For this review, take the finished solid that the model builds, in its own axes (mm). Face numbers are marked on the shaded views. A direction names the side the tool comes from. Round coordinates to 2 decimals unless told otherwise and drop trailing zeros. Loops run counter-clockwise (first coordinate to the right, second up) from the corner with the lowest first, then second, coordinate; pieces in that order, holes last. Notation, with made-up numbers: (19, 77) -> (39, 77) arc R30 ccw to (39, 109) -> close; hole circle Ø2 at (-21.5, 37). An arc over 180 degrees is marked (long way). One line per question, with ' | ' between items. Start each with the question number.
1. Consider section B-B (z = -89). Write out the cut boundary in (x, y).
2. Consider section A-A (x = 101). Write out the cut boundary in (y, z), and give its area (3 significant figures).
3. Consider section C-C (y = 9). Write out the cut boundary in (x, z), and give its area (3 significant figures).
4. For pin 1 Ø5 at (x, y) = (41.5, 128.5) entering from -Z; pin 2 Ø12 at (x, z) = (59.5, 27.5) entering from -Y; pin 3 Ø10 at (x, y) = (40, 102) entering from -Z, all flat-tipped, find the tip position at first contact; note any pin that passes through.
5. For the marked faces 1, 2, 3, 4 and 5, list the 3-axis set-ups (+Z, -Z, +X, -X, +Y, -Y) from which the entire face can be reached by the end or side of a thin tool; tool diameter is ignored.
6. Wall thickness on line 1 along X through (y, z) = (99.5, 60); line 2 along Y through (x, z) = (-52, -47): over which ranges is each line inside the solid? List them lowest first.
7. Consider section D-D (z = -6.5). Write out the cut boundary in (x, y), and give its area (3 significant figures).
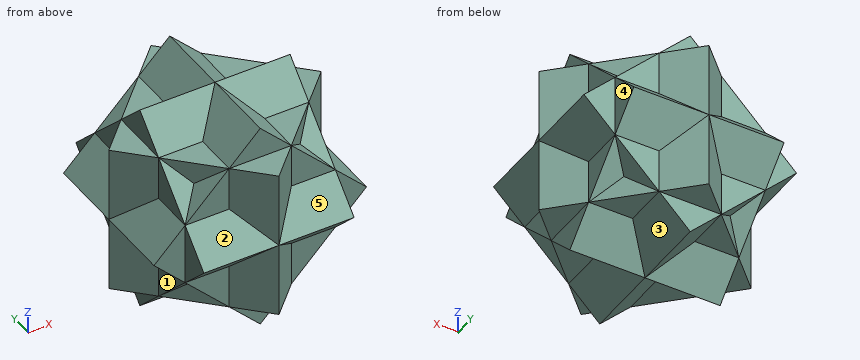
```python
from build123d import *

# Parameters (mm, degrees)
BOSS_EXTRUDE1_DEPTH = 113.704878
BOSS_EXTRUDE2_DEPTH = 113.704878
BOSS_EXTRUDE3_DEPTH = 113.704878


with BuildPart() as part:
    # Sketch3 → Boss-Extrude1 (new, symmetric)
    with BuildSketch(Plane.XY):
        Polygon((-160.802980576, 0), (0, 160.802980576), (160.802980576, 0), (0, -160.802980576), align=None)
    extrude(amount=BOSS_EXTRUDE1_DEPTH, both=True)

    # Sketch4 → Boss-Extrude2 (add, symmetric)
    with BuildSketch(Plane(origin=(0, 0, 0), x_dir=(1, 0, 0), z_dir=(0, 1, 0))):
        Polygon((-160.802980576, 0), (0, 160.802980576), (160.802980576, 0), (0, -160.802980576), align=None)
    extrude(amount=BOSS_EXTRUDE2_DEPTH, both=True)

    # Sketch5 → Boss-Extrude3 (add, symmetric)
    with BuildSketch(Plane(origin=(0, 0, 0), x_dir=(0, 0, -1), z_dir=(1, 0, 0))):
        Polygon((-160.802980576, 0), (0, 160.802980576), (160.802980576, 0), (0, -160.802980576), align=None)
    extrude(amount=BOSS_EXTRUDE3_DEPTH, both=True)


solid = part.part
```
Answer block:
1) outline: (-160.8, 0) -> (-113.7, -47.1) -> (-113.7, -71.8) -> (-89, -71.8) -> (-71.8, -89) -> (-71.8, -113.7) -> (-47.1, -113.7) -> (0, -160.8) -> (47.1, -113.7) -> (71.8, -113.7) -> (71.8, -89) -> (89, -71.8) -> (113.7, -71.8) -> (113.7, -47.1) -> (160.8, 0) -> (113.7, 47.1) -> (113.7, 71.8) -> (89, 71.8) -> (71.8, 89) -> (71.8, 113.7) -> (47.1, 113.7) -> (0, 160.8) -> (-47.1, 113.7) -> (-71.8, 113.7) -> (-71.8, 89) -> (-89, 71.8) -> (-113.7, 71.8) -> (-113.7, 47.1) -> close
2) outline: (-160.8, 0) -> (-113.7, -47.1) -> (-113.7, -59.8) -> (-101, -59.8) -> (-59.8, -101) -> (-59.8, -113.7) -> (-47.1, -113.7) -> (0, -160.8) -> (47.1, -113.7) -> (59.8, -113.7) -> (59.8, -101) -> (101, -59.8) -> (113.7, -59.8) -> (113.7, -47.1) -> (160.8, 0) -> (113.7, 47.1) -> (113.7, 59.8) -> (101, 59.8) -> (59.8, 101) -> (59.8, 113.7) -> (47.1, 113.7) -> (0, 160.8) -> (-47.1, 113.7) -> (-59.8, 113.7) -> (-59.8, 101) -> (-101, 59.8) -> (-113.7, 59.8) -> (-113.7, 47.1) -> close | area: 52,400 mm2
3) outline: (-160.8, 0) -> (-151.8, -9) -> (-151.8, -113.7) -> (-113.7, -113.7) -> (-113.7, -151.8) -> (-9, -151.8) -> (0, -160.8) -> (9, -151.8) -> (113.7, -151.8) -> (113.7, -113.7) -> (151.8, -113.7) -> (151.8, -9) -> (160.8, 0) -> (151.8, 9) -> (151.8, 113.7) -> (113.7, 113.7) -> (113.7, 151.8) -> (9, 151.8) -> (0, 160.8) -> (-9, 151.8) -> (-113.7, 151.8) -> (-113.7, 113.7) -> (-151.8, 113.7) -> (-151.8, 9) -> close | area: 86,700 mm2
4) pin 1: stops at z = -34.8 | pin 2: stops at y = -139.3 | pin 3: stops at z = -125.8
5) face 1: -Z, -X, -Y | face 2: +Z, -X, -Y | face 3: -Z, +X, +Y | face 4: +Z, -Z, +X, +Y | face 5: +Z, +X, -Y
6) line 1: x = -113.7 to 113.7 | line 2: y = -113.8 to 113.8
7) outline: (-160.8, 0) -> (-154.3, -6.5) -> (-154.3, -113.7) -> (-113.7, -113.7) -> (-113.7, -154.3) -> (-6.5, -154.3) -> (0, -160.8) -> (6.5, -154.3) -> (113.7, -154.3) -> (113.7, -113.7) -> (154.3, -113.7) -> (154.3, -6.5) -> (160.8, 0) -> (154.3, 6.5) -> (154.3, 113.7) -> (113.7, 113.7) -> (113.7, 154.3) -> (6.5, 154.3) -> (0, 160.8) -> (-6.5, 154.3) -> (-113.7, 154.3) -> (-113.7, 113.7) -> (-154.3, 113.7) -> (-154.3, 6.5) -> close | area: 88,800 mm2
